Could you check a few things on this model? Use its own coordinates, in mm. Give positions to 0.01 mm unless a question says otherwise; leave off trailing zeros. Order: outer loops, then holes, each group sorted by start corner. A loop starts at its lowest first (then second) coordinate and runs counter-clockwise, first axis right, second up.
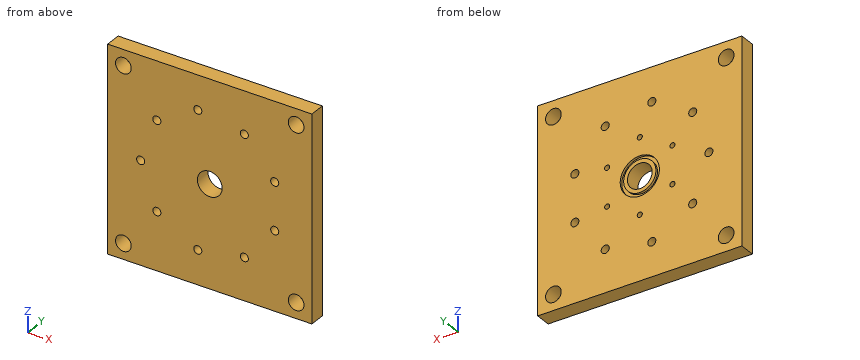
from build123d import *

# Parameters (mm, degrees)
SKETCH1_W           = 82.55
SKETCH1_H           = 82.55
BOSS_EXTRUDE1_DEPTH = 6.35
CUT_EXTRUDE1_REACH  = 8.35
SKETCH2_R           = 4.99999
SKETCH4_R           = 7.9248
SKETCH4_R_2         = 6.5278
CUT_EXTRUDE3_DEPTH  = 0.9779
SKETCH5_R           = 1.03251
CUT_EXTRUDE4_DEPTH  = 3.175
CIRPATTERN1_COUNT   = 6
SKETCH6_R           = 1.63195
CUT_EXTRUDE5_DEPTH  = 6.35
CIRPATTERN2_COUNT   = 9
CUT_EXTRUDE6_REACH  = 8.35
SKETCH7_R           = 3.175


with BuildPart() as part:
    # Sketch1 → Boss-Extrude1 (new body)
    with BuildSketch(Plane(origin=(0, 0, 0), x_dir=(1, 0, 0), z_dir=(0, 1, 0))):
        Rectangle(SKETCH1_W, SKETCH1_H)
    extrude(amount=BOSS_EXTRUDE1_DEPTH)

    # Sketch2 → Cut-Extrude1 (cut, up to next)
    with BuildSketch(Plane(origin=(0, 6.35, 0), x_dir=(1, 0, 0), z_dir=(0, 1, 0)), mode=Mode.PRIVATE) as cut_extrude1_sk1:
        Circle(SKETCH2_R)
    cut_extrude1_tool1 = extrude(cut_extrude1_sk1.sketch, amount=-CUT_EXTRUDE1_REACH, mode=Mode.PRIVATE) & part.part
    add(cut_extrude1_tool1.solids().sort_by_distance((0, 6.35, 0))[0], mode=Mode.SUBTRACT)

    # Sketch4 → Cut-Extrude3 (cut)
    with BuildSketch(Plane(origin=(0, 6.35, 0), x_dir=(1, 0, 0), z_dir=(0, 1, 0))):
        Circle(SKETCH4_R)
        Circle(SKETCH4_R_2, mode=Mode.SUBTRACT)
    extrude(amount=-CUT_EXTRUDE3_DEPTH, mode=Mode.SUBTRACT)

    # Sketch5 → Cut-Extrude4 (cut)
    with BuildSketch(Plane(origin=(0, 6.35, 0), x_dir=(1, 0, 0), z_dir=(0, 1, 0))):
        with Locations((0, -15.24)):
            Circle(SKETCH5_R)
    cut_extrude4 = extrude(amount=-CUT_EXTRUDE4_DEPTH, mode=Mode.SUBTRACT)

    # CirPattern1: Cut-Extrude4 ×6 about axis
    cirpattern1_axis = Axis((0, 0, 0), (0, 1, 0))
    for i in range(1, CIRPATTERN1_COUNT):
        add(cut_extrude4.rotate(cirpattern1_axis, i * 360 / CIRPATTERN1_COUNT), mode=Mode.SUBTRACT)

    # Sketch6 → Cut-Extrude5 (cut)
    with BuildSketch(Plane(origin=(0, 6.35, 0), x_dir=(1, 0, 0), z_dir=(0, 1, 0))):
        with Locations((13.97, -24.196749782)):
            Circle(SKETCH6_R)
    cut_extrude5 = extrude(amount=-CUT_EXTRUDE5_DEPTH, mode=Mode.SUBTRACT)

    # CirPattern2: Cut-Extrude5 ×9 about axis
    cirpattern2_axis = Axis((0, 0, 0), (0, 1, 0))
    for i in range(1, CIRPATTERN2_COUNT):
        add(cut_extrude5.rotate(cirpattern2_axis, i * 360 / CIRPATTERN2_COUNT), mode=Mode.SUBTRACT)

    # Sketch7 → Cut-Extrude6 (cut, up to next)
    with BuildSketch(Plane(origin=(0, 6.35, 0), x_dir=(1, 0, 0), z_dir=(0, 1, 0)), mode=Mode.PRIVATE) as cut_extrude6_sk1:
        with Locations((34.925, 34.925)):
            Circle(SKETCH7_R)
    cut_extrude6_tool1 = extrude(cut_extrude6_sk1.sketch, amount=-CUT_EXTRUDE6_REACH, mode=Mode.PRIVATE) & part.part
    add(cut_extrude6_tool1.solids().sort_by_distance((34.925, 6.35, -34.925))[0], mode=Mode.SUBTRACT)
    # Sketch7 → Cut-Extrude6 (cut, up to next)
    with BuildSketch(Plane(origin=(0, 6.35, 0), x_dir=(1, 0, 0), z_dir=(0, 1, 0)), mode=Mode.PRIVATE) as cut_extrude6_sk2:
        with Locations((34.925, -34.925)):
            Circle(SKETCH7_R)
    cut_extrude6_tool2 = extrude(cut_extrude6_sk2.sketch, amount=-CUT_EXTRUDE6_REACH, mode=Mode.PRIVATE) & part.part
    add(cut_extrude6_tool2.solids().sort_by_distance((34.925, 6.35, 34.925))[0], mode=Mode.SUBTRACT)
    # Sketch7 → Cut-Extrude6 (cut, up to next)
    with BuildSketch(Plane(origin=(0, 6.35, 0), x_dir=(1, 0, 0), z_dir=(0, 1, 0)), mode=Mode.PRIVATE) as cut_extrude6_sk3:
        with Locations((-34.925, -34.925)):
            Circle(SKETCH7_R)
    cut_extrude6_tool3 = extrude(cut_extrude6_sk3.sketch, amount=-CUT_EXTRUDE6_REACH, mode=Mode.PRIVATE) & part.part
    add(cut_extrude6_tool3.solids().sort_by_distance((-34.925, 6.35, 34.925))[0], mode=Mode.SUBTRACT)
    # Sketch7 → Cut-Extrude6 (cut, up to next)
    with BuildSketch(Plane(origin=(0, 6.35, 0), x_dir=(1, 0, 0), z_dir=(0, 1, 0)), mode=Mode.PRIVATE) as cut_extrude6_sk4:
        with Locations((-34.925, 34.925)):
            Circle(SKETCH7_R)
    cut_extrude6_tool4 = extrude(cut_extrude6_sk4.sketch, amount=-CUT_EXTRUDE6_REACH, mode=Mode.PRIVATE) & part.part
    add(cut_extrude6_tool4.solids().sort_by_distance((-34.925, 6.35, -34.925))[0], mode=Mode.SUBTRACT)


solid = part.part
Item 1: Please list where these lines run through material, in increasing order: line 1 along Z through (x, y) = (-27.94, 4.5) (3 decimals); line 2 along Z through (x, y) = (-20, 4.25) (3 decimals); line 3 along X through (y, z) = (4, -34) (3 decimals).
Findings:
line 1: z = -41.275 to -1.632, 1.632 to 41.275
line 2: z = -41.275 to -18.793, -17.126 to 17.126, 18.793 to 41.275
line 3: x = -41.275 to -37.962, -31.888 to 31.888, 37.962 to 41.275
Item 2: For pin 1 (2 mm diameter, centred on x = 26.26, z = -9.56, fed in from -Y), with a flat end and sliding along its axis, tell me the tip position at first contact or that it passes through.
Findings:
pin 1: passes through
Item 3: Imagine slicing it at A-A on z = 0. List the corners of the cut face in (x, y) for me (3 decimals).
Findings:
outline: (-41.275, 0) - (-29.572, 0) - (-29.572, 6.35) - (-41.275, 6.35) - close; (-26.308, 0) - (-5, 0) - (-5, 6.35) - (-6.528, 6.35) - (-6.528, 5.372) - (-7.925, 5.372) - (-7.925, 6.35) - (-26.308, 6.35) - close; (5, 0) - (41.275, 0) - (41.275, 6.35) - (7.925, 6.35) - (7.925, 5.372) - (6.528, 5.372) - (6.528, 6.35) - (5, 6.35) - close
Item 4: Imagine slicing it at B-B on x = 0. List the corners of the cut face in (y, z) for me (3 decimals).
Findings:
outline: (0, -41.275) - (6.35, -41.275) - (6.35, -16.273) - (3.175, -16.273) - (3.175, -14.207) - (6.35, -14.207) - (6.35, -7.925) - (5.372, -7.925) - (5.372, -6.528) - (6.35, -6.528) - (6.35, -5) - (0, -5) - close; (0, 5) - (6.35, 5) - (6.35, 6.528) - (5.372, 6.528) - (5.372, 7.925) - (6.35, 7.925) - (6.35, 14.207) - (3.175, 14.207) - (3.175, 16.273) - (6.35, 16.273) - (6.35, 41.275) - (0, 41.275) - close
Item 5: Imagine slicing it at C-C on z = -18.5. List the corners of the cut face in (x, y) for me (3 decimals), then the cut area to 3 significant figures.
Findings:
outline: (-41.275, 0) - (-22.943, 0) - (-22.943, 6.35) - (-41.275, 6.35) - close; (-19.863, 0) - (41.275, 0) - (41.275, 6.35) - (-19.863, 6.35) - close
area: 505 mm2
